For this review, take the finished solid that the model builds, in its own axes (mm). A direction names the side the tool comes from. Give positions to 0.01 mm unless a question says otherwise; leave off trailing zeros. Order: outer loops, then holes, each group sorted by start corner. A loop starts at its lowest first (then second) coordinate and runs counter-clockwise, first axis right, second up. Notation, with made-up numbers: (27.25, -16.75) - (60.25, -16.75) arc R17 ccw to (60.25, 1.25) - close; hole circle Ø8 at (74.5, -16). An arc over 180 degrees is marked (long way). One line per item, written item: value.
```python
from build123d import *

# Parameters (mm, degrees)
SKETCH2_W               = 170.18
SKETCH2_H               = 228.6
SKETCH2_W_2             = 119.38
SKETCH2_H_2             = 177.8
BOSS_EXTRUDE1_DEPTH     = 25.4
CUT_EXTRUDE1_REACH      = 146.741
SKETCH3_R               = 3.175
MIRROR2_COPY_1_REACH    = 146.741
MIRROR2_COPY_1_SKETCH_R = 3.175


with BuildPart() as part:
    # Sketch2 → Boss-Extrude1 (new body)
    with BuildSketch(Plane(origin=(0, 0, 0), x_dir=(1, 0, 0), z_dir=(0, 1, 0))):
        Rectangle(SKETCH2_W, SKETCH2_H)
        Rectangle(SKETCH2_W_2, SKETCH2_H_2, mode=Mode.SUBTRACT)
    extrude(amount=BOSS_EXTRUDE1_DEPTH)

    # Sketch3 → Cut-Extrude1 (cut, up to next)
    with BuildSketch(Plane(origin=(0, 25.4, 0), x_dir=(1, 0, 0), z_dir=(0, 1, 0)), mode=Mode.PRIVATE) as cut_extrude1_sk1:
        with Locations(Location((-66.04, 69.85, 0), (0, 0, 270))):
            Circle(SKETCH3_R)
    cut_extrude1_tool1 = extrude(cut_extrude1_sk1.sketch, amount=-CUT_EXTRUDE1_REACH, mode=Mode.PRIVATE) & part.part
    # Sketch3 → Cut-Extrude1 (cut, up to next)
    with BuildSketch(Plane(origin=(0, 25.4, 0), x_dir=(1, 0, 0), z_dir=(0, 1, 0)), mode=Mode.PRIVATE) as cut_extrude1_sk2:
        with Locations(Location((-40.64, 95.25, 0), (0, 0, 270))):
            Circle(SKETCH3_R)
    cut_extrude1_tool2 = extrude(cut_extrude1_sk2.sketch, amount=-CUT_EXTRUDE1_REACH, mode=Mode.PRIVATE) & part.part
    cut_extrude1_1 = cut_extrude1_tool1.solids().sort_by_distance((-66.04, 25.4, -69.85))[0]
    add(cut_extrude1_1, mode=Mode.SUBTRACT)
    cut_extrude1_2 = cut_extrude1_tool2.solids().sort_by_distance((-40.64, 25.4, -95.25))[0]
    add(cut_extrude1_2, mode=Mode.SUBTRACT)
    cut_extrude1 = cut_extrude1_1 + cut_extrude1_2  # Cut-Extrude1 as one shape, for the pattern or mirror that repeats it

    # Mirror1: Cut-Extrude1 across plane
    add(cut_extrude1.mirror(Plane(origin=(0, 0, 0), x_dir=(0, 0, 1), z_dir=(1, 0, 0))), mode=Mode.SUBTRACT)

    # Mirror2: Cut-Extrude1 across plane
    add(cut_extrude1.mirror(Plane.XY), mode=Mode.SUBTRACT)

    # Mirror2 copy 1 sketch → Mirror2 copy 1 (cut, up to next)
    with BuildSketch(Plane(origin=(0, 25.4, 0), x_dir=(-1, 0, 0), z_dir=(0, 1, 0)), mode=Mode.PRIVATE) as mirror2_copy_1_sk1:
        with Locations(Location((-66.04, 69.85, 0), (0, 0, 270))):
            Circle(MIRROR2_COPY_1_SKETCH_R)
    mirror2_copy_1_tool1 = extrude(mirror2_copy_1_sk1.sketch, amount=-MIRROR2_COPY_1_REACH, mode=Mode.PRIVATE) & part.part
    # Mirror2 copy 1 sketch → Mirror2 copy 1 (cut, up to next)
    with BuildSketch(Plane(origin=(0, 25.4, 0), x_dir=(-1, 0, 0), z_dir=(0, 1, 0)), mode=Mode.PRIVATE) as mirror2_copy_1_sk2:
        with Locations(Location((-40.64, 95.25, 0), (0, 0, 270))):
            Circle(MIRROR2_COPY_1_SKETCH_R)
    mirror2_copy_1_tool2 = extrude(mirror2_copy_1_sk2.sketch, amount=-MIRROR2_COPY_1_REACH, mode=Mode.PRIVATE) & part.part
    add(mirror2_copy_1_tool1.solids().sort_by_distance((66.04, 25.4, 69.85))[0], mode=Mode.SUBTRACT)
    add(mirror2_copy_1_tool2.solids().sort_by_distance((40.64, 25.4, 95.25))[0], mode=Mode.SUBTRACT)


solid = part.part
```
(1) Take a section at D-D (y = 2.5). Give the number of separate pieces and of enclosed holes in the cut face, then the cut area to 3 significant figures.
Answers below:
separate pieces: 1
enclosed holes: 9
area: 17,400 mm^2
(2) Take a section at B-B (z = -69.85). Write out the cut boundary in (x, y) (3 decimals), then the cut area to 3 significant figures.
Answers below:
outline: (-85.09, 0) - (-69.215, 0) - (-69.215, 25.4) - (-85.09, 25.4) - close; (-62.865, 0) - (-59.69, 0) - (-59.69, 25.4) - (-62.865, 25.4) - close; (59.69, 0) - (62.865, 0) - (62.865, 25.4) - (59.69, 25.4) - close; (69.215, 0) - (85.09, 0) - (85.09, 25.4) - (69.215, 25.4) - close
area: 968 mm^2
(3) Take a section at C-C (z = -95.25). Write out the cut boundary in (x, y) (3 decimals), then the cut area to 3 significant figures.
Answers below:
outline: (-85.09, 0) - (-43.815, 0) - (-43.815, 25.4) - (-85.09, 25.4) - close; (-37.465, 0) - (37.465, 0) - (37.465, 25.4) - (-37.465, 25.4) - close; (43.815, 0) - (85.09, 0) - (85.09, 25.4) - (43.815, 25.4) - close
area: 4,000 mm^2
(4) Take a section at A-A (x = -66.04). Write out the cut boundary in (y, z) (3 decimals), then the cut area to 3 significant figures.
Answers below:
outline: (0, -114.3) - (25.4, -114.3) - (25.4, -73.025) - (0, -73.025) - close; (0, -66.675) - (25.4, -66.675) - (25.4, 66.675) - (0, 66.675) - close; (0, 73.025) - (25.4, 73.025) - (25.4, 114.3) - (0, 114.3) - close
area: 5,480 mm^2
(5) Draft analysis for pull direction X (two halves, no side actions). For faces 1 (the face through (62.89, 12.88, -70.26)), 2 (the face through (-1, 13, 114.3)), 3 (the face through (-85.09, 13, 2)), state which applies: pulls with the +X half, pulls with the -X half, needs draft (parallel to the pull), parting line crosses it, or undercut.
Answers below:
face 1: undercut
face 2: needs draft
face 3: pulls with the -X half
(6) Machinability: for faces 4 (the face through (-1, 13, -88.9)), 5 (the face through (85.09, 13, 2)), which of the approach directions +Z, -Z, +X, -X, +Y, -Y give a long, thin tool a straight path to every point of the face, cutting with its end or side? Answer none if there is none.
Answers below:
face 4: +Y, -Y
face 5: +Z, -Z, +X, +Y, -Y
(7) Wall thickness on line 1 (X direction, y = 18.5, z = -95.25) (3 decimals); line 2 (X direction, y = 18.5, z = 69.85) (3 decimals); line 3 (Z direction, x = 66.04, y = 17.75) (3 decimals): over which ranges is each line inside the solid? List them lowest first. Write a range as from..to.
Answers below:
line 1: x = -85.09..-43.815, -37.465..37.465, 43.815..85.09
line 2: x = -85.09..-69.215, -62.865..-59.69, 59.69..62.865, 69.215..85.09
line 3: z = -114.3..-73.025, -66.675..66.675, 73.025..114.3
